The listing builds one solid part. Answer for the finished solid, in the listing's coordinates (mm). A direction names the side the tool comes from. Coordinates: 2 decimals unless noted, no trailing zeros. Order: outer loops, then holes, each group sorted by start corner. A loop starts at its lowest first (then second) coordinate and runs counter-clockwise, first axis right, second up. Notation, with made-up numbers: (29.25, 4) -> (52.25, 4) arc R28 ccw to (52.25, 24) -> close; hole circle Ø8 at (2, 75.5). An arc over 180 degrees is marked (long way). Return JSON: item names as keys, results as strings.
```python
from build123d import *

# Parameters (mm, degrees)
SKETCH1_W           = 215
SKETCH1_H           = 168
SKETCH1_R           = 3
SKETCH1_R_2         = 2
BOSS_EXTRUDE1_DEPTH = 21
CHAMFER1_SIZE       = 4
SKETCH2_R           = 9.5
CUT_EXTRUDE1_DEPTH  = 13
SKETCH4_R           = 5
CUT_EXTRUDE2_DEPTH  = 6.5


with BuildPart() as part:
    # Sketch1 → Boss-Extrude1 (new body)
    with BuildSketch(Plane(origin=(0, 0, 0), x_dir=(1, 0, 0), z_dir=(0, 1, 0))):
        with Locations((107.5, 84)):
            Rectangle(SKETCH1_W, SKETCH1_H)
        with Locations((150, 118)):
            Circle(SKETCH1_R, mode=Mode.SUBTRACT)
        with Locations((65, 118)):
            Circle(SKETCH1_R, mode=Mode.SUBTRACT)
        with Locations((65, 48)):
            Circle(SKETCH1_R, mode=Mode.SUBTRACT)
        with Locations((150, 48)):
            Circle(SKETCH1_R, mode=Mode.SUBTRACT)
        with Locations((20, 15.5)):
            Circle(SKETCH1_R_2, mode=Mode.SUBTRACT)
        with Locations((195, 15.5)):
            Circle(SKETCH1_R_2, mode=Mode.SUBTRACT)
    extrude(amount=BOSS_EXTRUDE1_DEPTH)

    # Chamfer1
    chamfer1_edges = [part.edges().sort_by_distance(p)[0] for p in [
        (215, 21, -84),
        (107.5, 21, -168),
        (0, 21, -84),
        (107.5, 21, 0),
    ]]
    chamfer(chamfer1_edges, length=CHAMFER1_SIZE)

    # Sketch2 → Cut-Extrude1 (cut)
    with BuildSketch(Plane.XZ):
        with Locations((65, -48)):
            Circle(SKETCH2_R)
        with Locations((150, -48)):
            Circle(SKETCH2_R)
        with Locations((65, -118)):
            Circle(SKETCH2_R)
        with Locations((150, -118)):
            Circle(SKETCH2_R)
    extrude(amount=-CUT_EXTRUDE1_DEPTH, mode=Mode.SUBTRACT)

    # Sketch4 → Cut-Extrude2 (cut)
    with BuildSketch(Plane.XZ):
        with Locations((20, -15.5)):
            Circle(SKETCH4_R)
        with Locations((195, -15.5)):
            Circle(SKETCH4_R)
    extrude(amount=-CUT_EXTRUDE2_DEPTH, mode=Mode.SUBTRACT)


solid = part.part
```
Item 1: Find the intervals of material crossed by probe 1 along X at (y, z) = (15.75, -48); probe 2 along Z at (x, y) = (65, 3.75); probe 3 along Z at (x, y) = (65, 15.25), in increasing order.
Answer list:
{"probe 1": "0 to 62, 68 to 147, 153 to 215", "probe 2": "-168 to -127.5, -108.5 to -57.5, -38.5 to 0", "probe 3": "-168 to -121, -115 to -51, -45 to 0"}
Item 2: The part is cut by section A-A on y = 9. Determine the outline of the cut face in (x, z).
Answer list:
{"outline": "(0, -168) -> (215, -168) -> (215, 0) -> (0, 0) -> close; hole circle Ø4 at (20, -15.5); hole circle Ø19 at (65, -118); hole circle Ø19 at (65, -48); hole circle Ø19 at (150, -118); hole circle Ø19 at (150, -48); hole circle Ø4 at (195, -15.5)"}
Item 3: Which of the six approach directions +Z, -Z, +X, -X, +Y, -Y give full straight-line access (tool end or side, diameter ignored) to faces 4 (the flat face through (106, 8, 0)), 5 (the cylindrical face through (140.51, 6.41, -47.58))?
Answer list:
{"face 4": "+Z, +X, -X, +Y, -Y", "face 5": "-Y"}
Item 4: Determine the mould class of faces 1 (the flat face through (106, 8, -168)), 2 (the flat face through (62.76, 13, -45.76)), 3 (the flat face through (215, 8, -83)) for opening direction Z: pulls with the +Z half, pulls with the -Z half, needs draft (parallel to the pull), parting line crosses it, or undercut.
Answer list:
{"face 1": "pulls with the -Z half", "face 2": "undercut", "face 3": "needs draft"}
Item 5: Flat-ended cylindrical pins translate along their axes: pin 1 (5 mm diameter, centred on x = 125, y = 18.5, fed in from +Z); pin 2 (5 mm diameter, centred on x = 195, z = -15.5, fed in from -Y); pin 3 (5.5 mm diameter, centred on x = 154, z = -121, fed in from -Y). Find the tip coordinate at first contact, or state that the pin passes through.
Answer list:
{"pin 1": "z = 0", "pin 2": "y = 6.5", "pin 3": "y = 13"}
Item 6: The part is cut by section C-C on z = -48. Determine the outline of the cut face in (x, y).
Answer list:
{"outline": "(0, 0) -> (55.5, 0) -> (55.5, 13) -> (62, 13) -> (62, 21) -> (4, 21) -> (0, 17) -> close; (68, 13) -> (74.5, 13) -> (74.5, 0) -> (140.5, 0) -> (140.5, 13) -> (147, 13) -> (147, 21) -> (68, 21) -> close; (153, 13) -> (159.5, 13) -> (159.5, 0) -> (215, 0) -> (215, 17) -> (211, 21) -> (153, 21) -> close"}
Item 7: The part is cut by section B-B on x = 65. Determine the outline of the cut face in (y, z).
Answer list:
{"outline": "(0, -168) -> (17, -168) -> (21, -164) -> (21, -121) -> (13, -121) -> (13, -127.5) -> (0, -127.5) -> close; (0, -108.5) -> (13, -108.5) -> (13, -115) -> (21, -115) -> (21, -51) -> (13, -51) -> (13, -57.5) -> (0, -57.5) -> close; (0, -38.5) -> (13, -38.5) -> (13, -45) -> (21, -45) -> (21, -4) -> (17, 0) -> (0, 0) -> close"}
